from build123d import *

# Parameters (mm, degrees)
BOSS_EXTRUDE1_DEPTH = 1.57
SKETCH4_R           = 0.8
CUT_EXTRUDE1_DEPTH  = 2.57


with BuildPart() as part:
    # Sketch2 → Boss-Extrude1 (new body)
    with BuildSketch(Plane.XY):
        Polygon((-14, -55.500103029), (-14, -51.671572877), (-18.878667627, -46.792905249), (-6.278214078, -34.1924517), (7.156814765, -47.627480542), (19.177630045, -35.606665262), (5, -21.429035217), (5, -5), (59, -5), (59, -8.204229809), (37.000000001, -36.704229808), (37.000000001, -49.491817554), (30.165562087, -55.500103029), align=None)
    extrude(amount=BOSS_EXTRUDE1_DEPTH)

    # Sketch4 → Cut-Extrude1 (cut, through all)
    with BuildSketch(Plane.XY.offset(1.57)):
        with Locations((39.999798764, -7.5)):
            Circle(SKETCH4_R)
        with Locations((39.999898107, -27.999885516)):
            Circle(SKETCH4_R)
        with Locations((24.000063681, -52.999991481)):
            Circle(SKETCH4_R)
        with Locations((6.3681e-05, -52.999991481)):
            Circle(SKETCH4_R)
    extrude(amount=-CUT_EXTRUDE1_DEPTH, mode=Mode.SUBTRACT)


solid = part.part
The model under review builds one solid part; all positions refer to its coordinate system, in mm. A direction names the side the tool comes from. Round coordinates to 2 decimals unless told otherwise and drop trailing zeros. Write each loop counter-clockwise with the first axis right and the second up, starting at its lowest first coordinate (ties: lowest second). Pieces come first, ordered by that corner, then holes. Notation, with made-up numbers: M 52,17.5 L 60,17.5 A8 cw 60,25.5 Z; hole C 0,83 d1. An arc over 180 degrees is marked long. Use a Markdown table: item, result. Add a question column.
Q1. We need section D-D, the plane x = -12. State the section outline as (y, z) points.
Q2. We need section C-C, the plane y = -17.5. State the section outline as (x, z) points, plus the area to 3 significant figures.
Q3. Machinability: for faces 1 (the face through (8, -55.5, 1)), 2 (the face through (-14, -54, 1)), 3 (the face through (37, -43, 1)), 4 (the face through (5, -13, 1)), 5 (the face through (13.083, -41.701, 0.774)), which of the approach directions +Z, -Z, +X, -X, +Y, -Y give a long, thin tool a straight path to every point of the face, cutting with its end or side? Answer none if there is none.
Q4. The part is to be moulded in two halves that separate along X. For faces 6 (the face through (48.154, -22.255, 0.774)), 7 (the face through (21, -30, 0)), 8 (the face through (0.37, -53.71, 0.8)), say which applies: pulls with the +X half, pulls with the -X half, needs draft (parallel to the pull), parting line crosses it, or undercut.
Q5. We need section B-B, the plane z = 1.1. State the section outline as (x, y) points.
Q6. To check wall thickness, follow line 1 (Y direction, x = 16, z = 0.3); line 2 (Y direction, x = 0.5, z = 0.15); line 3 (X direction, y = -50, z = 1.4). State the ranges of each line that lie inside material, in increasing order.
Q7. We need section A-A, the plane x = 11.5. State the section outline as (y, z) points.
Q8. Insertion check: pin 1 (0.5 mm diameter, centred on y = -40.5, z = 1, fed in from +X); pin 2 (1 mm diameter, centred on x = 40, y = -28, fed in from -Z); pin 3 (3 mm diameter, centred on x = -3.5, y = -39.5, fed in from -Z); pin 4 (0.8 mm diameter, centred on y = -13, z = 0.5, fed in from -X). Each pin has a flat end and moves straight along its axis. Give the tip position at first contact, or say it passes through.
Findings below:
| question | item | result |
|---|---|---|
| 1 | outline | M -55.5,0 L -39.91,0 L -39.91,1.57 L -55.5,1.57 Z |
| 2 | outline | M 5,0 L 51.82,0 L 51.82,1.57 L 5,1.57 Z |
| 2 | area | 73.5 mm² |
| 3 | face 1 | +Z, -Z, +X, -X, -Y |
| 3 | face 2 | +Z, -Z, -X, -Y |
| 3 | face 3 | +Z, -Z, +X, -Y |
| 3 | face 4 | +Z, -Z, -X, +Y |
| 3 | face 5 | +Z, -Z |
| 4 | face 6 | pulls with the +X half |
| 4 | face 7 | needs draft |
| 4 | face 8 | undercut |
| 5 | outline | M -18.88,-46.79 L -14,-51.67 L -14,-55.5 L 30.17,-55.5 L 37,-49.49 L 37,-36.7 L 59,-8.2 L 59,-5 L 5,-5 L 5,-21.43 L 19.18,-35.61 L 7.16,-47.63 L -6.28,-34.19 Z; hole C 0,-53 d1.6; hole C 24,-53 d1.6; hole C 40,-28 d1.6; hole C 40,-7.5 d1.6 |
| 6 | line 1 | y = -55.5 to -38.78, -32.43 to -5 |
| 6 | line 2 | y = -55.5 to -53.62, -52.38 to -40.97 |
| 6 | line 3 | x = -15.67 to 36.42 |
| 7 | outline | M -55.5,0 L -43.28,0 L -43.28,1.57 L -55.5,1.57 Z; M -27.93,0 L -5,0 L -5,1.57 L -27.93,1.57 Z |
| 8 | pin 1 | stops at x = 37 |
| 8 | pin 2 | passes through |
| 8 | pin 3 | stops at z = 0 |
| 8 | pin 4 | stops at x = 5 |
